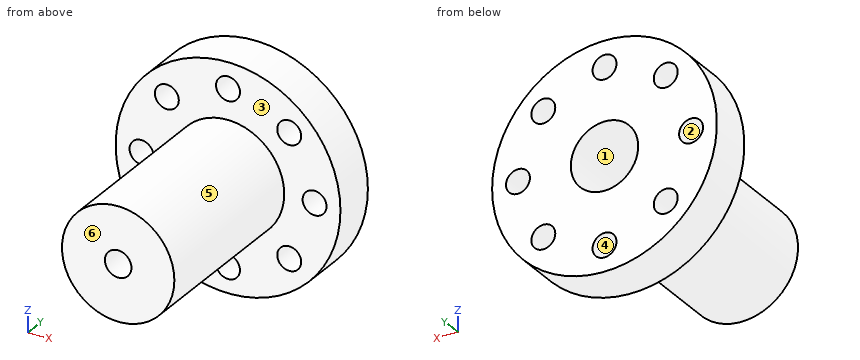
```python
from build123d import *

# Parameters (mm, degrees)
CIRPATTERN1_COUNT  = 8
SKETCH5_R          = 3.81
CUT_EXTRUDE1_DEPTH = 20.828
SKETCH6_R          = 1.4986
CUT_EXTRUDE2_DEPTH = 5.572


with BuildPart() as part:
    # Sketch1 → Revolve1 (revolve)
    with BuildSketch(Plane.XY):
        Polygon((12.7, 0), (0, 0), (0, -25.4), (6.35, -25.4), (6.35, -5.08), (12.7, -5.08), align=None)
    revolve(axis=Axis((0, 0, 0), (0, -1, 0)))

    # Sketch4 → #6-32 Tapped Hole1 (revolve, cut)
    with BuildSketch(Plane(origin=(0, 0, 9.779), x_dir=(0, 0, 1), z_dir=(1, 0, 0))):
        Polygon((0, 0), (0, 10.21069403), (1.35255, 9.398), (1.35255, 0), align=None)
    f_6_32_tapped_hole1 = revolve(axis=Axis((0, 6.35, 9.779), (0, -1, 0)), mode=Mode.SUBTRACT)

    # CirPattern1: #6-32 Tapped Hole1 ×8 about axis
    cirpattern1_axis = Axis((0, 0, 0), (0, 1, 0))
    for i in range(1, CIRPATTERN1_COUNT):
        add(f_6_32_tapped_hole1.rotate(cirpattern1_axis, i * 360 / CIRPATTERN1_COUNT), mode=Mode.SUBTRACT)

    # Sketch5 → Cut-Extrude1 (cut)
    with BuildSketch(Plane(origin=(0, 0, 0), x_dir=(1, 0, 0), z_dir=(0, 1, 0))):
        Circle(SKETCH5_R)
    extrude(amount=-CUT_EXTRUDE1_DEPTH, mode=Mode.SUBTRACT)

    # Sketch6 → Cut-Extrude2 (cut, through all)
    with BuildSketch(Plane(origin=(0, -20.828, 0), x_dir=(1, 0, 0), z_dir=(0, 1, 0))):
        Circle(SKETCH6_R)
    extrude(amount=-CUT_EXTRUDE2_DEPTH, mode=Mode.SUBTRACT)


solid = part.part
```
Could you check a few things on this model? Use its own coordinates, in mm. Face numbers are marked on the shaded views. A direction names the side the tool comes from. Coordinates: 2 decimals unless noted, no trailing zeros. Write each loop counter-clockwise with the first axis right and the second up, starting at its lowest first coordinate (ties: lowest second). Pieces come first, ordered by that corner, then holes. Notation, with made-up numbers: (-10, -4.5) -> (33, -4.5) arc R19 cw to (33, 9.5) -> close; hole circle Ø11 at (61, 13.25). An arc over 180 degrees is marked (long way). Return JSON: item names as keys, results as strings.
(1) We'd pull the mould along Z, two halves only. Please class the marked faces 4, 5 and 6: +Z half, -Z half, draft (parallel to the pull), parting line (faces both ways), or undercut.
Numbers:
{"face 4": "undercut", "face 5": "parting line", "face 6": "draft"}
(2) I'm going to push flat-ended pins straight in: pin 1 (2 mm diameter, centred on x = 6.91, z = 6.91, fed in from +Y) (1 decimal); pin 2 (6 mm diameter, centred on x = 0, z = 0, fed in from +Y); pin 3 (1.5 mm diameter, centred on x = 4.5, y = -16.5, fed in from +Z); pin 4 (10 mm diameter, centred on x = -6.5, y = -4.5, fed in from +Z). Where does each tip first touch, or does it pass through?
Numbers:
{"pin 1": "passes through", "pin 2": "stops at y = -20.83", "pin 3": "stops at z = 5.12", "pin 4": "stops at z = 12.61"}
(3) Imagine slicing it at B-B, the plane z = 0. Please give me the cut outline in (x, y), then the cut area to 3 significant figures.
Numbers:
{"outline": "(-12.7, -5.08) -> (-11.13, -5.08) -> (-11.13, 0) -> (-12.7, 0) -> close; (-8.43, -5.08) -> (-6.35, -5.08) -> (-6.35, -25.4) -> (-1.5, -25.4) -> (-1.5, -20.83) -> (-3.81, -20.83) -> (-3.81, 0) -> (-8.43, 0) -> close; (1.5, -25.4) -> (6.35, -25.4) -> (6.35, -5.08) -> (8.43, -5.08) -> (8.43, 0) -> (3.81, 0) -> (3.81, -20.83) -> (1.5, -20.83) -> close; (11.13, -5.08) -> (12.7, -5.08) -> (12.7, 0) -> (11.13, 0) -> close", "area": "187 mm2"}
(4) I need wall thicknesses on L1, parallel to Z at x = 0, y = -9; L2, parallel to X at y = -3, z = -6; L3, parallel to X at y = -16.5, z = -3. Which ranges of each line are inside material? Lowest first, please.
Numbers:
{"L1": "z = -6.35 to -3.81, 3.81 to 6.35", "L2": "x = -11.19 to -7.91, -5.92 to 5.92, 7.91 to 11.19", "L3": "x = -5.6 to -2.35, 2.35 to 5.6"}
(5) Which directions (+Z, -Z, +X, -X, +Y, -Y) give clear straight access to the entire face, cutting with the end or side of a thin tool? Please do the marked faces 1, 2 and 3.
Numbers:
{"face 1": "+Y", "face 2": "+Y, -Y", "face 3": "-Y"}
(6) Imagine slicing it at C-C, the plane x = 6.75. Please give me the cut outline in (y, z).
Numbers:
{"outline": "(-5.08, -10.76) -> (0, -10.76) -> (0, -8.26) -> (-5.08, -8.26) -> close; (-5.08, -5.57) -> (0, -5.57) -> (0, 5.57) -> (-5.08, 5.57) -> close; (-5.08, 8.26) -> (0, 8.26) -> (0, 10.76) -> (-5.08, 10.76) -> close"}
(7) Imagine slicing it at D-D, the plane y = -10.75. Please give me the cut outline in (x, z), then the cut area to 3 significant figures.
Numbers:
{"outline": "circle Ø12.7 at (0, 0); hole circle Ø7.62 at (0, 0)", "area": "81.1 mm2"}
(8) Imagine slicing it at A-A, the plane x = 0. Please give me the cut outline in (y, z).
Numbers:
{"outline": "(-25.4, -6.35) -> (-5.08, -6.35) -> (-5.08, -8.43) -> (0, -8.43) -> (0, -3.81) -> (-20.83, -3.81) -> (-20.83, -1.5) -> (-25.4, -1.5) -> close; (-25.4, 1.5) -> (-20.83, 1.5) -> (-20.83, 3.81) -> (0, 3.81) -> (0, 8.43) -> (-5.08, 8.43) -> (-5.08, 6.35) -> (-25.4, 6.35) -> close; (-5.08, -12.7) -> (0, -12.7) -> (0, -11.13) -> (-5.08, -11.13) -> close; (-5.08, 11.13) -> (0, 11.13) -> (0, 12.7) -> (-5.08, 12.7) -> close"}
